Source: CAD feature listing. Evaluate the final solid. Frame: model axes, mm. Round coordinates to 2 decimals unless told otherwise and drop trailing zeros. Write each loop counter-clockwise with the first axis right and the second up, starting at its lowest first coordinate (ties: lowest second). Pieces come first, ordered by that corner, then holes. Notation, with made-up numbers: M 29.25,71.5 L 62.25,71.5 A26 cw 62.25,94.5 Z; hole C 62.5,37 d8. An arc over 180 degrees is marked long. Use a Markdown table: item, result.
```python
from build123d import *

# Parameters (mm, degrees)
F0_R     = 10
F0_R_2   = 5
F1_DEPTH = 6.35


with BuildPart() as f1:
    # F0 (on Top) → F1 (new body)
    with BuildSketch(Plane.XY):
        with BuildLine():
            Line((15, 22), (15, 80))
            Line((15, 80), (-15, 80))
            Line((-15, 80), (-15, -20))
            Line((-15, -20), (85, -20))
            Line((85, -20), (85, 20))
            Line((85, 20), (17, 20))
            ThreePointArc((17, 20), (13.585786, 18.585786), (15, 22))
        make_face()
        Circle(F0_R, mode=Mode.SUBTRACT)
        Polygon((25, -5.773503), (35, 11.547005), (45, -5.773503), align=None, mode=Mode.SUBTRACT)
        with Locations((70, 0)):
            Circle(F0_R_2, mode=Mode.SUBTRACT)
    extrude(amount=F1_DEPTH)


solid = f1.part
```
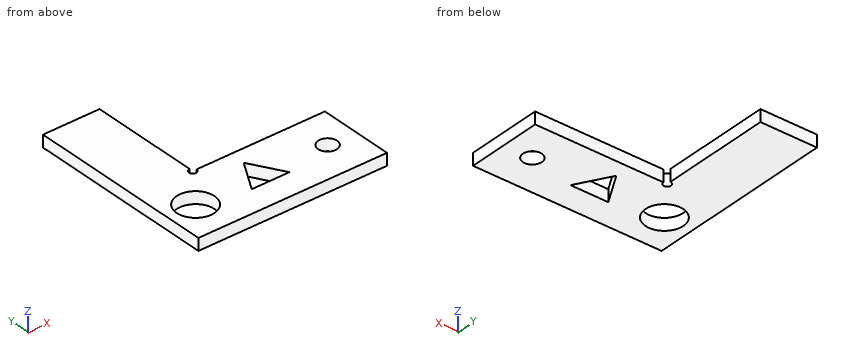
Q1. Section A-A on x = 0. Return loops of the section in (y, z).
Results are:
| item | result |
|---|---|
| outline | M -20,0 L -10,0 L -10,6.35 L -20,6.35 Z; M 10,0 L 80,0 L 80,6.35 L 10,6.35 Z |
Q2. Line query: L1, parallel to Y at x = 0, z = 3; L2, parallel to Y at x = 70, z = 2.25; L3, parallel to X at y = 9, z = 3. Output: solid intervals per line, ascending.
Results are:
| item | result |
|---|---|
| L1 | -20 to -10, 10 to 80 |
| L2 | -20 to -5, 5 to 20 |
| L3 | -15 to -4.36, 4.36 to 33.53, 36.47 to 85 |
Q3. First-contact query: pin 1 Ø3 at (x, z) = (33, 2.5) entering from +Y; pin 2 Ø1 at (y, z) = (60, 3.5) entering from +X. Flat tips, straight axial feed; report the tip coordinate or a pass-through.
Results are:
| item | result |
|---|---|
| pin 1 | y = 20 |
| pin 2 | x = 15 |
Q4. Section D-D on x = 70. Return loops of the section in (y, z), plus the area to 4 significant figures.
Results are:
| item | result |
|---|---|
| outline | M -20,0 L -5,0 L -5,6.35 L -20,6.35 Z; M 5,0 L 20,0 L 20,6.35 L 5,6.35 Z |
| area | 190.5 mm^2 |
Q5. Section B-B on z = 4.75. Return loops of the section in (x, y).
Results are:
| item | result |
|---|---|
| outline | M -15,-20 L 85,-20 L 85,20 L 17,20 A2 cw long 15,22 L 15,80 L -15,80 Z; hole C 0,0 d20; hole M 25,-5.77 L 45,-5.77 L 35,11.55 Z; hole C 70,0 d10 |
Q6. Section C-C on y = 0. Return loops of the section in (x, z), plus the area to 3 significant figures.
Results are:
| item | result |
|---|---|
| outline | M -15,0 L -10,0 L -10,6.35 L -15,6.35 Z; M 10,0 L 28.33,0 L 28.33,6.35 L 10,6.35 Z; M 41.67,0 L 65,0 L 65,6.35 L 41.67,6.35 Z; M 75,0 L 85,0 L 85,6.35 L 75,6.35 Z |
| area | 360 mm^2 |
